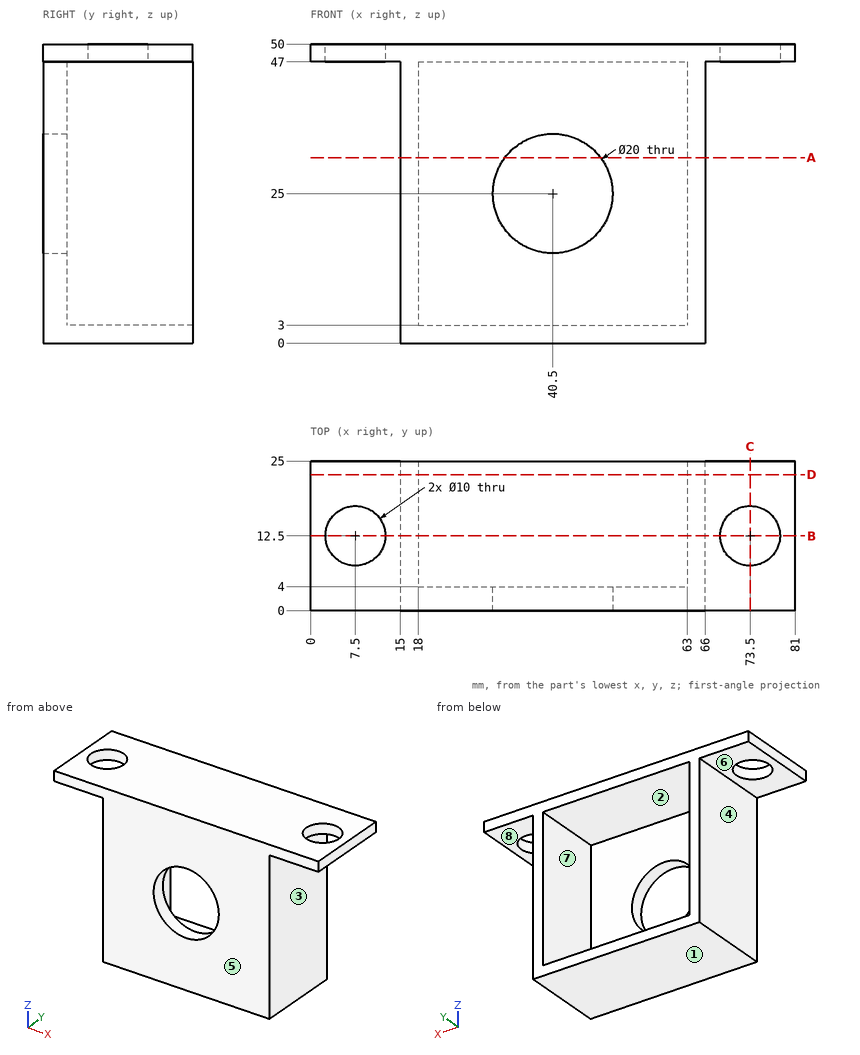
For this review, use the dimensioned drawing (mm, ordinates from the lowest corner) and the shaded views. A direction names the side the tool comes from. Coordinates: 2 decimals unless noted, no trailing zeros. Write each loop counter-clockwise with the first axis right and the second up, starting at its lowest first coordinate (ties: lowest second). Pieces come first, ordered by that corner, then holes. Notation, with made-up numbers: (22, -15.75) - (44, -15.75) arc R11 ccw to (44, -7.75) - close; hole circle Ø11 at (3.25, -37). An arc over 180 degrees is marked (long way). Answer as a JSON object with one key per item and string values. Group by question number.
1. Add section B-B (y = 12.5). Give the boundary of the cut face in (x, z).
2. Mouldability with a two-part tool opening along X and no side actions: class the marked faces 1, 2, 3 and 4 as pulls with the +X half, pulls with the -X half, needs draft (parallel to the pull), parting line crosses it, or undercut.
3. Add section A-A (z = 31). Give the boundary of the cut face in (x, y), plus the area to 3 significant figures.
4. Clearance check with flat-ended pins moving along their axes: pin 1 Ø1.5 at (y, z) = (8.5, 18) entering from +X; pin 2 Ø12.5 at (y, z) = (8, 15) entering from -X; pin 3 Ø4.5 at (x, y) = (6.5, 17.5) entering from -Z. State where each tip first meets the part, or that it passes through.
5. Add section D-D (y = 22.75). Give the boundary of the cut face in (x, z), plus the area to 3 significant figures.
6. Add section C-C (x = 73.5). Give the boundary of the cut face in (y, z).
7. Machinability: for the marked faces 5, 6, 7 and 8, which of the approach directions +Z, -Z, +X, -X, +Y, -Y give a long, thin tool a straight path to every point of the face, cutting with its end or side? Answer none if there is none.
8. To check wall thickness, follow probe 1 along X at (y, z) = (17, 30.5); probe 2 along Z at (x, y) = (40.5, 2.85); probe 3 along Z at (x, y) = (50, 17.5). State the ranges of each line that lie inside material, in increasing order.
Findings:
{
 "1": {"outline": "(0, 47) - (2.5, 47) - (2.5, 50) - (0, 50) - close; (12.5, 47) - (15, 47) - (15, 0) - (66, 0) - (66, 47) - (68.5, 47) - (68.5, 50) - (12.5, 50) - close; (78.5, 47) - (81, 47) - (81, 50) - (78.5, 50) - close; hole (18, 3) - (63, 3) - (63, 47) - (18, 47) - close"},
 "2": {"face 1": "needs draft", "face 2": "undercut", "face 3": "pulls with the +X half", "face 4": "pulls with the -X half"},
 "3": {"outline": "(15, 0) - (32.5, 0) - (32.5, 4) - (18, 4) - (18, 25) - (15, 25) - close; (48.5, 0) - (66, 0) - (66, 25) - (63, 25) - (63, 4) - (48.5, 4) - close", "area": "266 mm²"},
 "4": {"pin 1": "x = 66", "pin 2": "x = 15", "pin 3": "z = 47"},
 "5": {"outline": "(0, 47) - (15, 47) - (15, 0) - (66, 0) - (66, 47) - (81, 47) - (81, 50) - (0, 50) - close; hole (18, 3) - (63, 3) - (63, 47) - (18, 47) - close", "area": "660 mm²"},
 "6": {"outline": "(0, 47) - (7.5, 47) - (7.5, 50) - (0, 50) - close; (17.5, 47) - (25, 47) - (25, 50) - (17.5, 50) - close"},
 "7": {"face 5": "+Z, -Z, +X, -X, -Y", "face 6": "-Z, -X, +Y, -Y", "face 7": "+Y", "face 8": "-Z, +X, +Y, -Y"},
 "8": {"probe 1": "15 to 18, 63 to 66", "probe 2": "0 to 15, 35 to 50", "probe 3": "0 to 3, 47 to 50"}
}
